Verification items for the finished model (mm, model axes). Coordinates: 2 decimals unless noted, no trailing zeros. Order: outer loops, then holes, each group sorted by start corner. A loop starts at its lowest first (then second) coordinate and runs counter-clockwise, first axis right, second up. Notation, with made-up numbers: (-15.75, 42.25) -> (17.25, 42.25) arc R37 cw to (17.25, 80.25) -> close; hole circle Ø5 at (4.25, 88.25). An arc over 180 degrees is marked (long way). Use CSV: the item, a comma, the result in double quotes. Start each with the question number.
1) Scan lines: line 1 along X through (y, z) = (-7, -2); line 2 along X through (y, z) = (-0.25, 10); line 3 along Z through (x, y) = (5, -4). Record each from-to range of solid material in increasing order.
2) Sectioned sample at A-A on x = 8. Record the boundary of the cut face in (y, z), then the cut area to 3 significant figures.
3) Sectioned sample at C-C on y = -2.75. Record the boundary of the cut face in (x, z).
4) Go/stop test with flat-tipped pins: pin 1 (1.5 mm diameter, centred on y = -6, z = -2.5, fed in from +X); pin 2 (3 mm diameter, centred on y = -5.5, z = -16, fed in from -X); pin 3 (1 mm diameter, centred on y = -4.5, z = -1, fed in from -X). Record where each tip stops, or that it passes through.
5) Sectioned sample at B-B on z = 1.5. Record the boundary of the cut face in (x, y).
from build123d import *

# Parameters (mm, degrees)
F1_DEPTH = 15
F2_SIZE  = 2
F3_SCALE = 0.5


with BuildPart() as f1:
    # F0 (on Front) → F1 (new body)
    with BuildSketch(Plane.XZ):
        Polygon((-0.1495843466, -46.6474431687), (40.472662979, 23.1941777401), (-40.3230786324, 23.4532654285), align=None)
    extrude(amount=F1_DEPTH)

    # F2
    f2_edges = [f1.edges().sort_by_distance(p)[0] for p in [
        (0.074792, -15, 23.323722),
        (20.161539, -15, -11.726633),
        (-20.236331, -15, -11.597089),
    ]]
    chamfer(f2_edges, length=F2_SIZE)


with BuildPart() as f1_1:
    # F3: moved
    add(f1.part.scale(F3_SCALE))


solid = f1_1.part
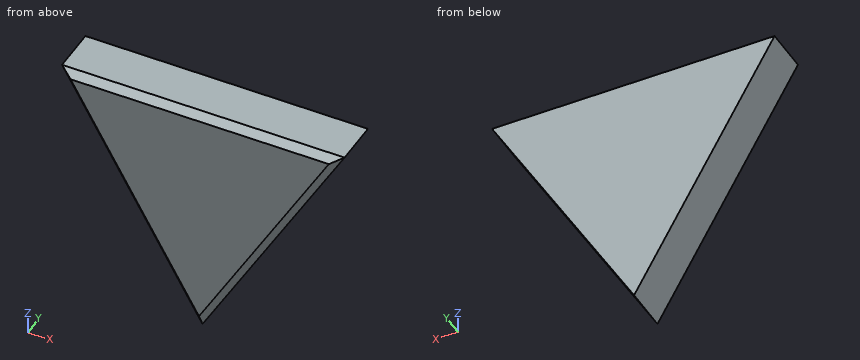
Answers follow:
1,line 1,"x = -11.72 to 11.75"
1,line 2,"x = -19.17 to 19.31"
1,line 3,"z = -14.6 to 11.65"
2,outline,"(-7.5, -7.45) -> (-6.5, -9.44) -> (0, -9.44) -> (0, 11.64) -> (-6.5, 11.64) -> (-7.5, 10.64) -> close"
2,area,"157 mm²"
3,outline,"(-20.16, 11.73) -> (-0.07, -23.32) -> (20.24, 11.6) -> close"
4,pin 1,"stops at x = 12.47"
4,pin 2,"stops at x = -5.13"
4,pin 3,"stops at x = -13.15"
5,outline,"(-14.3, -6.5) -> (-13.15, -7.5) -> (13.21, -7.5) -> (14.36, -6.5) -> (14.36, 0) -> (-14.3, 0) -> close"
